The model under review builds one solid part; all positions refer to its coordinate system, in mm. A direction names the side the tool comes from. Give positions to 0.01 mm unless a question says otherwise; leave off trailing zeros. Loops run counter-clockwise (first coordinate to the right, second up) from the corner with the lowest first, then second, coordinate; pieces in that order, holes last. Notation, with made-up numbers: (77, 86) - (83, 86) arc R25 cw to (83, 104) - close; hole circle Ø1 at (42, 10). An arc over 180 degrees is marked (long way). Answer as a JSON object with one key per item and string values.
from build123d import *

# Parameters (mm, degrees)
SKETCH2_R           = 1.25
BOSS_EXTRUDE1_DEPTH = 1.25


with BuildPart() as part:
    # Sketch2 → Boss-Extrude1 (new body)
    with BuildSketch(Plane.XY):
        with BuildLine():
            Line((0.279648542, 3.739558355), (-25, 5.63))
            Line((-25, 5.63), (-45.347946147, 3.733822904))
            ThreePointArc((-45.347946147, 3.733822904), (-48.75, 0), (-45.347946147, -3.733822904))
            Line((-45.347946147, -3.733822904), (-25, -5.63))
            Line((-25, -5.63), (-7.098436577, -4.377631434))
            ThreePointArc((-7.098436577, -4.377631434), (-4.815909482, -5.147037966), (-3.75577728, -7.309914769))
            Line((-3.75577728, -7.309914769), (-3.12422272, -17.690085231))
            ThreePointArc((-3.12422272, -17.690085231), (0, -20.63), (3.12422272, -17.690085231))
            Line((3.12422272, -17.690085231), (3.747638192, -0.133071355))
            ThreePointArc((3.747638192, -0.133071355), (2.793577424, 2.501684467), (0.279648542, 3.739558355))
        make_face()
        Circle(SKETCH2_R, mode=Mode.SUBTRACT)
        with Locations((0, -17.5)):
            Circle(SKETCH2_R, mode=Mode.SUBTRACT)
        with Locations((-45, 0)):
            Circle(SKETCH2_R, mode=Mode.SUBTRACT)
        with Locations((-25, 0)):
            Circle(SKETCH2_R, mode=Mode.SUBTRACT)
        with Locations((-39.37, 1.25)):
            Circle(SKETCH2_R, mode=Mode.SUBTRACT)
    extrude(amount=BOSS_EXTRUDE1_DEPTH)


solid = part.part
Q1. Clearance check with a flat-ended pin moving along its axis: pin 1 Ø1.5 at (x, y) = (-45, 0) entering from +Z. State where the tip first meets the part, or that it passes through.
Results:
{"pin 1": "passes through"}
Q2. Consider section D-D, the plane x = -21. State the section outline as (y, z) points.
Results:
{"outline": "(-5.35, 0) - (5.33, 0) - (5.33, 1.25) - (-5.35, 1.25) - close"}
Q3. Consider section C-C, the plane x = -39.37. State the section outline as (y, z) points, plus the area to 3 significant figures.
Results:
{"outline": "(-4.29, 0) - (0, 0) - (0, 1.25) - (-4.29, 1.25) - close; (2.5, 0) - (4.29, 0) - (4.29, 1.25) - (2.5, 1.25) - close", "area": "7.60 mm^2"}
Q4. Consider section A-A, the plane z = 0.85. State the section outline as (x, y) points, plus the area to 3 significant figures.
Results:
{"outline": "(-45.35, -3.73) - (-25, -5.63) - (-7.1, -4.38) arc R3.13 cw to (-3.76, -7.31) - (-3.12, -17.69) arc R3.13 ccw to (3.12, -17.69) - (3.75, -0.13) arc R3.75 ccw to (0.28, 3.74) - (-25, 5.63) - (-45.35, 3.73) arc R3.75 ccw to start; hole circle Ø2.5 at (-45, 0); hole circle Ø2.5 at (-39.37, 1.25); hole circle Ø2.5 at (-25, 0); hole circle Ø2.5 at (0, -17.5); hole circle Ø2.5 at (0, 0)", "area": "558 mm^2"}
Q5. For faces 4 (the face through (-38.18, 1.63, 0.62)), 5 (the face through (-16, -5, 1)), list the 3-axis set-ups (+Z, -Z, +X, -X, +Y, -Y) from which the entire face can be reached by the end or side of a thin tool; tool diameter is ignored.
Results:
{"face 4": "+Z, -Z", "face 5": "+Z, -Z, -Y"}
Q6. The part is to be moulded in two halves that separate along Y. For faces 1 (the face through (-0.27, -1.22, 0.62)), 2 (the face through (-35, 4.7, 0.6)), 3 (the face through (-35.32, -4.67, 0.62)), say which applies: +Y half, -Y half, draft (parallel to the pull), parting line (faces both ways), or undercut.
Results:
{"face 1": "undercut", "face 2": "+Y half", "face 3": "-Y half"}
Q7. Consider section B-B, the plane y = -5. State the section outline as (x, z) points.
Results:
{"outline": "(-31.76, 0) - (-15.99, 0) - (-15.99, 1.25) - (-31.76, 1.25) - close; (-5, 0) - (3.57, 0) - (3.57, 1.25) - (-5, 1.25) - close"}
Q8. To check wall thickness, follow probe 1 along Y at (x, z) = (0, 0.3); probe 2 along Y at (x, z) = (-25, 0.8); probe 3 along Y at (x, z) = (-24, 0.3). State the ranges of each line that lie inside material, in increasing order. Write a range as [from, to].
Results:
{"probe 1": "y = [-20.63, -18.75], [-16.25, -1.25], [1.25, 3.76]", "probe 2": "y = [-5.63, -1.25], [1.25, 5.63]", "probe 3": "y = [-5.56, -0.75], [0.75, 5.56]"}
